Can you work these out from the model? Positions are in its coordinate system, mm. Give positions to 0.01 mm unless a question says otherwise; leave off trailing zeros. Loops run counter-clockwise (first coordinate to the right, second up) from the corner with the lowest first, then second, coordinate; pieces in that order, holes last. Notation, with made-up numbers: (6.5, 27) -> (47.5, 27) arc R37 cw to (47.5, 63) -> close; hole circle Ø8 at (-1, -24). An arc over 180 degrees is marked (long way). One line per question, with ' | ' between items.
from build123d import *

# Parameters (mm, degrees)
BOSS_EXTRUDE1_DEPTH = 46.0375
SKETCH3_R           = 2.7051
CUT_EXTRUDE1_DEPTH  = 38.1
CUT_EXTRUDE2_START  = -38.1
SKETCH4_R           = 2.7051
CUT_EXTRUDE2_DEPTH  = 38.1


with BuildPart() as part:
    # Sketch2 → Boss-Extrude1 (new, symmetric)
    with BuildSketch(Plane.XY):
        Polygon((0, 6.415804866), (-5.55625, 3.207902433), (-5.55625, -3.207902433), (0, -6.415804866), (5.55625, -3.207902433), (5.55625, 3.207902433), align=None)
    extrude(amount=BOSS_EXTRUDE1_DEPTH, both=True)

    # Sketch3 → Cut-Extrude1 (cut)
    with BuildSketch(Plane.XY.offset(46.0375)):
        Circle(SKETCH3_R)
    extrude(amount=-CUT_EXTRUDE1_DEPTH, mode=Mode.SUBTRACT)

    # Sketch4 → Cut-Extrude2 (cut)
    with BuildSketch(Plane(origin=(0, 0, -46.0375), x_dir=(-1, 0, 0), z_dir=(0, 0, -1)).offset(CUT_EXTRUDE2_START)):
        with Locations(Location((0, 0, 0), (0, 0, 180))):
            Circle(SKETCH4_R)
    extrude(amount=CUT_EXTRUDE2_DEPTH, mode=Mode.SUBTRACT)


solid = part.part
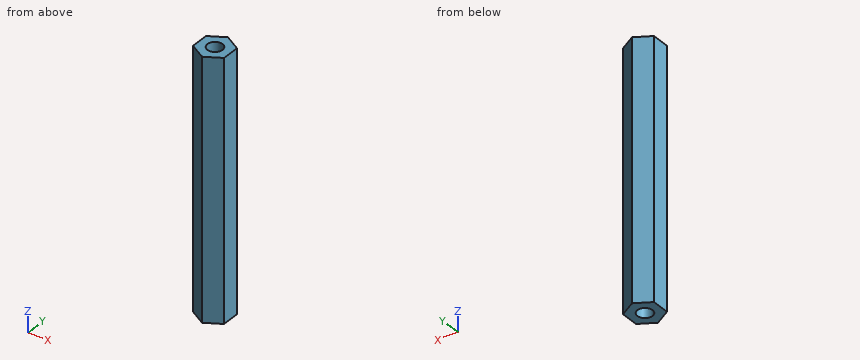
Q1. If we section it at A-A (z = -27): Write out the boundary of the cut face in (x, y).
Entries:
outline: (-5.56, -3.21) -> (0, -6.42) -> (5.56, -3.21) -> (5.56, 3.21) -> (0, 6.42) -> (-5.56, 3.21) -> close; hole circle Ø5.41 at (0, 0)
Q2. If I drill on probe 1 along Y at (x, z) = (0, 33); probe 2 along Z at (x, y) = (-1.75, 0.5); probe 3 along Y at (x, z) = (-0.25, -27), over which ranges is the centre line in solid material (lowest first)? Write a range as from..to.
Entries:
probe 1: -6.42..-2.71, 2.71..6.42 | probe 2: -7.94..7.94 | probe 3: -6.27..-2.69, 2.69..6.27
Q3. For pin 1 Ø1.5 at (y, z) = (4.5, -11.5) entering from -X; pin 2 Ø5 at (x, y) = (0, 0) entering from -Z; pin 3 Ø4.5 at (x, y) = (0, 0) entering from +Z, each with a flat end and sliding along its axis, tell me the tip position at first contact or that it passes through.
Entries:
pin 1: x = -4.62 | pin 2: z = -7.94 | pin 3: z = 7.94
Q4. If we section it at C-C (z = -1): Write out the boundary of the cut face in (x, y).
Entries:
outline: (-5.56, -3.21) -> (0, -6.42) -> (5.56, -3.21) -> (5.56, 3.21) -> (0, 6.42) -> (-5.56, 3.21) -> close
Q5. If we section it at B-B (y = 0): Write out the boundary of the cut face in (x, z).
Entries:
outline: (-5.56, -46.04) -> (-2.71, -46.04) -> (-2.71, -7.94) -> (2.71, -7.94) -> (2.71, -46.04) -> (5.56, -46.04) -> (5.56, 46.04) -> (2.71, 46.04) -> (2.71, 7.94) -> (-2.71, 7.94) -> (-2.71, 46.04) -> (-5.56, 46.04) -> close
